For this review, take the finished solid that the model builds, in its own axes (mm). Face numbers are marked on the shaded views. A direction names the side the tool comes from. Round coordinates to 2 decimals unless told otherwise and drop trailing zeros. Write each loop counter-clockwise with the first axis right and the second up, starting at its lowest first coordinate (ties: lowest second). Pieces come first, ordered by that corner, then holes. Notation, with made-up numbers: (-19.5, 30) -> (7.5, 30) arc R24 ccw to (7.5, 64) -> close; hole circle Ø5 at (87, 49). An arc over 180 degrees is marked (long way). Write item = value, one per line. Start each with the question number.
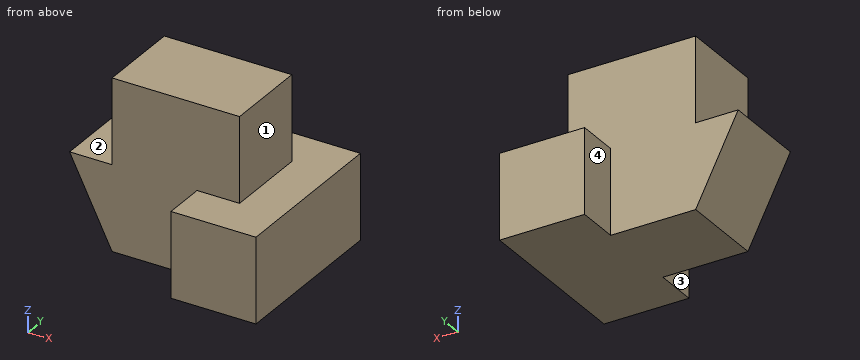
```python
from build123d import *

# Parameters (mm, degrees)
F0_W     = 50
F0_H     = 40
F1_DEPTH = 40
F2_W     = 10
F2_H     = 20
F3_DEPTH = 50.001
F4_W     = 30
F4_H     = 10
F5_DEPTH = 20.001
F6_W     = 10
F6_H     = 20
F7_DEPTH = 20
F8_W     = 10
F8_H     = 20
F9_DEPTH = 30.001


with BuildPart() as f1:
    # F0 (on Front) → F1 (new body)
    with BuildSketch(Plane.XZ):
        with Locations((25, 20)):
            Rectangle(F0_W, F0_H)
    extrude(amount=F1_DEPTH)

    # F2 (on face) → F3 (cut, through all)
    with BuildSketch(Plane(origin=(0, 0, 0), x_dir=(0, -1, 0), z_dir=(-1, 0, 0))):
        with Locations((5, 30)):
            Rectangle(F2_W, F2_H)
        with Locations((35, 30)):
            Rectangle(F2_W, F2_H)
    extrude(amount=-F3_DEPTH, mode=Mode.SUBTRACT)

    # F4 (on face) → F5 (cut, through all)
    with BuildSketch(Plane.XY.offset(20)):
        with Locations((15, -5)):
            Rectangle(F4_W, F4_H)
        with Locations((15, -35)):
            Rectangle(F4_W, F4_H)
    extrude(amount=-F5_DEPTH, mode=Mode.SUBTRACT)

    # F6 (on face) → F7 (cut, through all)
    with BuildSketch(Plane.XY.offset(40)):
        with Locations((45, -20)):
            Rectangle(F6_W, F6_H)
    extrude(amount=-F7_DEPTH, mode=Mode.SUBTRACT)

    # F8 (on face) → F9 (cut, through all)
    with BuildSketch(Plane.XZ.offset(30)):
        Polygon((10, 0), (0, 20), (0, 0), align=None)
        with Locations((5, 30)):
            Rectangle(F8_W, F8_H)
    extrude(amount=-F9_DEPTH, mode=Mode.SUBTRACT)


solid = f1.part
```
1. Wall thickness on L1, parallel to Y at x = 8, z = 11; L2, parallel to X at y = -33, z = 2; L3, parallel to Z at x = 43, y = -26: over which ranges is each line inside the solid? List them lowest first. Write a range as from..to.
2. Consider section D-D, the plane x = 26.5. Give the boundary of the cut face in (y, z).
3. Clearance check with flat-ended pins moving along their axes: pin 1 Ø8 at (y, z) = (-4, 5.5) entering from -X; pin 2 Ø5 at (x, y) = (4.5, -23) entering from +Z; pin 3 Ø5 at (x, z) = (7.5, 6) entering from -Y. State where each tip first meets the part, or that it passes through.
4. Consider section B-B, the plane x = 38. Give the boundary of the cut face in (y, z), then the cut area to 3 significant figures.
5. Machinability: for the marked faces 1, 2, 3 and 4, which of the approach directions +Z, -Z, +X, -X, +Y, -Y give a long, thin tool a straight path to every point of the face, cutting with its end or side? Answer none if there is none.
6. Consider section A-A, the plane y = -24.5. Give the boundary of the cut face in (x, z).
7. Consider section C-C, the plane z = 32. Give the boundary of the cut face in (x, y).
Outcome:
q1.L1 = -30..-10
q1.L2 = 30..50
q1.L3 = 0..20
q2.outline = (-30, 0) -> (-10, 0) -> (-10, 40) -> (-30, 40) -> close
q3.pin_1 = 30
q3.pin_2 = 20
q3.pin_3 = -30
q4.outline = (-40, 0) -> (0, 0) -> (0, 20) -> (-10, 20) -> (-10, 40) -> (-30, 40) -> (-30, 20) -> (-40, 20) -> close
q4.area = 1,200 mm2
q5.face_1 = +Z, +X, +Y, -Y
q5.face_2 = +Z, -X, +Y, -Y
q5.face_3 = +Z, -Z, -X, -Y
q5.face_4 = +Z, -Z, -X, +Y
q6.outline = (0, 20) -> (10, 0) -> (50, 0) -> (50, 20) -> (40, 20) -> (40, 40) -> (10, 40) -> (10, 20) -> close
q7.outline = (10, -30) -> (40, -30) -> (40, -10) -> (10, -10) -> close
